Read the model definition and answer for the solid it produces. Units are mm, in the model's axes. A direction names the side the tool comes from. Round coordinates to 2 decimals unless told otherwise and drop trailing zeros. Order: outer loops, then holes, each group sorted by start corner. A loop starts at its lowest first (then second) coordinate and runs counter-clockwise, first axis right, second up. Notation, with made-up numbers: (-27.5, 49.5) - (-21.5, 49.5) arc R19 cw to (-21.5, 83.5) - close; hole circle Ø8 at (-34.5, 54). An arc over 180 degrees is marked (long way). Answer as a JSON object with one key per item and string values. Group by question number.
Q1. The mould has two halves that part along X. Classify faces 1 (the flat face through (221.81, 31.22, 95.69)), 2 (the flat face through (190.5, 32, 96)), 3 (the flat face through (286, -6.35, 16)): pulls with the +X half, pulls with the -X half, needs draft (parallel to the pull), parting line crosses it, or undercut.
Q2. A tool of negligible diameter and unlimited length cuts with its end or side. For faces 4 (the flat face through (127, 31, 96)), 5 (the flat face through (285, -51, 31.75)), 6 (the flat face through (95, -6.35, 96)), 7 (the flat face through (95.25, -1, 16)), from which of +Z, -Z, +X, -X, +Y, -Y can it reach the whole face along a straight path? Write none if from no direction.
Q3. A cutting plane is placed at C-C on x = 203. Determine the outline of the cut face in (y, z), and give its area (3 significant figures).
Q4. A cutting plane is placed at A-A on z = 110. Determine the outline of the cut face in (x, y), and give its area (3 significant figures).
Q5. Consider line 1 (X direction, y = -20, z = 22.5); line 2 (X direction, y = 87, z = 26); line 3 (Z direction, x = 84, y = -16). Determine where each line is inside the solid, lowest interval first.
Q6. A cutting plane is placed at B-B on y = -75. Determine the outline of the cut face in (x, z).
Q7. Given pin 1 Ø4 at (x, y) = (68.5, -25.5) entering from +Z; pin 2 Ø19 at (x, z) = (162, 93) entering from -Y; pin 3 Ø20.5 at (y, z) = (82, 108) entering from +X, each flat-ended and moving along its own axis, determine where each tip first touches the part or whether it passes through.
Q8. A cutting plane is placed at D-D on y = 18.5. Determine the outline of the cut face in (x, z).
```python
from build123d import *

# Parameters (mm, degrees)
F1_DEPTH = 95.25
F2_W     = 63.5
F2_H     = 31.75
F3_DEPTH = 101.6
F5_START = -63.5
F4_W     = 63.5
F4_H     = 127
F5_DEPTH = 127
F7_START = -63.5
F7_DEPTH = 76.2


with BuildPart() as f1:
    # F0 (on Front) → F1 (new body, symmetric)
    with BuildSketch(Plane.XZ):
        Polygon((0, 63.5), (0, 0), (95.25, 0), (95.25, 31.75), (158.75, 31.75), (158.75, 0), (254, 0), (254, 31.75), (317.5, 31.75), (317.5, 63.5), align=None)
    extrude(amount=F1_DEPTH, both=True)

    # F2 (on face) → F3 (join)
    with BuildSketch(Plane(origin=(0, 95.25, 0), x_dir=(-1, 0, 0), z_dir=(0, 1, 0))):
        with Locations((-285.75, 15.875)):
            Rectangle(F2_W, F2_H)
    extrude(amount=-F3_DEPTH)

    # F4 (on face) → F5 (join)
    with BuildSketch(Plane.XZ.offset(95.25).offset(F5_START)):
        with Locations((31.75, 127)):
            Rectangle(F4_W, F4_H)
    extrude(amount=-F5_DEPTH)

    # F6 (on face) → F7 (join)
    with BuildSketch(Plane.XY.offset(190.5).offset(F7_START)):
        Polygon((254, 95.25), (63.5, 95.25), (63.5, -6.35), (127, -6.35), (127, 69.85), (190.5, 69.85), (190.5, -6.35), (254, 69.85), align=None)
    extrude(amount=-F7_DEPTH)


solid = f1.part
```
Result set:
{
 "1": {"face 1": "pulls with the +X half", "face 2": "undercut", "face 3": "needs draft"},
 "2": {"face 4": "+Z, -Y", "face 5": "-Z, +X, -Y", "face 6": "+Z, +X, -Y", "face 7": "-Z, +Y, -Y"},
 "3": {"outline": "(-95.25, 0) - (95.25, 0) - (95.25, 127) - (8.65, 127) - (8.65, 63.5) - (-95.25, 63.5) - close", "area": "17,600 mm²"},
 "4": {"outline": "(0, -31.75) - (63.5, -31.75) - (63.5, -6.35) - (127, -6.35) - (127, 69.85) - (190.5, 69.85) - (190.5, -6.35) - (254, 69.85) - (254, 95.25) - (0, 95.25) - close", "area": "20,200 mm²"},
 "5": {"line 1": "x = 0 to 95.25, 158.75 to 254", "line 2": "x = 0 to 95.25, 158.75 to 317.5", "line 3": "z = 0 to 63.5"},
 "6": {"outline": "(0, 0) - (95.25, 0) - (95.25, 31.75) - (158.75, 31.75) - (158.75, 0) - (254, 0) - (254, 31.75) - (317.5, 31.75) - (317.5, 63.5) - (0, 63.5) - close"},
 "7": {"pin 1": "stops at z = 63.5", "pin 2": "stops at y = 69.85", "pin 3": "stops at x = 254"},
 "8": {"outline": "(0, 0) - (95.25, 0) - (95.25, 31.75) - (158.75, 31.75) - (158.75, 0) - (317.5, 0) - (317.5, 63.5) - (211.21, 63.5) - (211.21, 127) - (190.5, 127) - (190.5, 63.5) - (127, 63.5) - (127, 127) - (63.5, 127) - (63.5, 190.5) - (0, 190.5) - close"}
}
